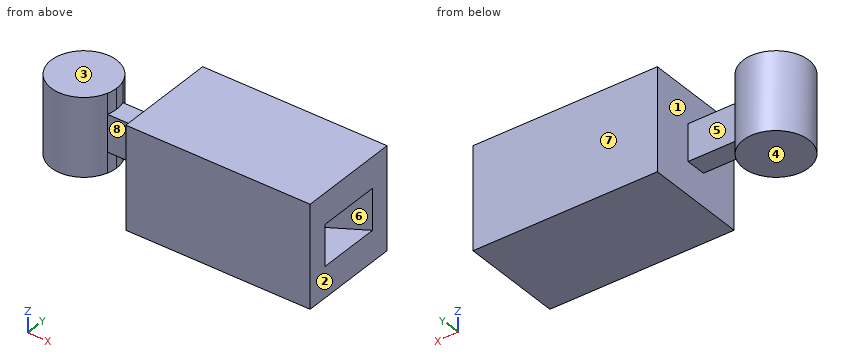
```python
from build123d import *

# Parameters (mm, degrees)
F1_DEPTH = 12.5
F2_DEPTH = 10
F3_DEPTH = 4.5
F4_DEPTH = 9.5
F5_DEPTH = 5


with BuildPart() as f1:
    # F0 (on Top) → F1 (new body, symmetric)
    with BuildSketch(Plane.XY):
        with BuildLine():
            Line((22.5, 12.5), (-22.5, 12.5))
            Line((-22.5, 12.5), (-22.5, 2.5))
            Line((-22.5, 2.5), (-22.5, -2.5))
            Line((-22.5, -2.5), (-22.5, -12.5))
            Line((-22.5, -12.5), (22.5, -12.5))
            Line((22.5, -12.5), (22.5, -7.75))
            Line((22.5, -7.75), (14.5, -3))
            ThreePointArc((14.5, -3), (-1.952987, 0), (14.5, 3))
            Line((14.5, 3), (22.5, 7.75))
            Line((22.5, 7.75), (22.5, 12.5))
        make_face()
        with BuildLine():
            ThreePointArc((15.047013, 0), (14.909142, 1.524731), (14.5, 3))
            ThreePointArc((14.5, 3), (-1.952987, 0), (14.5, -3))
            ThreePointArc((14.5, -3), (14.909142, -1.524731), (15.047013, 0))
        make_face()
        Polygon((22.5, -7.75), (22.5, -3), (14.5, -3), align=None)
        with BuildLine():
            Line((22.5, -3), (22.5, 3))
            Line((22.5, 3), (14.5, 3))
            ThreePointArc((14.5, 3), (14.909142, 1.524731), (15.047013, 0))
            ThreePointArc((15.047013, 0), (14.909142, -1.524731), (14.5, -3))
            Line((14.5, -3), (22.5, -3))
        make_face()
        Polygon((22.5, 3), (22.5, 7.75), (14.5, 3), align=None)
    extrude(amount=F1_DEPTH, both=True)

    # F0 (on Top) → F2 (cut, symmetric)
    with BuildSketch(Plane.XY):
        with BuildLine():
            ThreePointArc((15.047013, 0), (14.909142, 1.524731), (14.5, 3))
            ThreePointArc((14.5, 3), (-1.952987, 0), (14.5, -3))
            ThreePointArc((14.5, -3), (14.909142, -1.524731), (15.047013, 0))
        make_face()
    extrude(amount=F2_DEPTH, both=True, mode=Mode.SUBTRACT)

    # F0 (on Top) → F3 (join, symmetric)
    with BuildSketch(Plane.XY):
        with BuildLine():
            Line((-22.5, -2.5), (-22.5, 2.5))
            Line((-22.5, 2.5), (-34.5, 2.5))
            ThreePointArc((-34.5, 2.5), (-34.200142, 1.265951), (-34.099342, 0))
            ThreePointArc((-34.099342, 0), (-34.200142, -1.265951), (-34.5, -2.5))
            Line((-34.5, -2.5), (-22.5, -2.5))
        make_face()
    extrude(amount=F3_DEPTH, both=True)

    # F0 (on Top) → F4 (join, symmetric)
    with BuildSketch(Plane.XY):
        with BuildLine():
            ThreePointArc((-34.099342, 0), (-34.200142, 1.265951), (-34.5, 2.5))
            ThreePointArc((-34.5, 2.5), (-50.099342, 0), (-34.5, -2.5))
            ThreePointArc((-34.5, -2.5), (-34.200142, -1.265951), (-34.099342, 0))
        make_face()
    extrude(amount=F4_DEPTH, both=True)

    # F0 (on Top) → F5 (cut, symmetric)
    with BuildSketch(Plane.XY):
        Polygon((22.5, 3), (22.5, 7.75), (14.5, 3), align=None)
        with BuildLine():
            Line((22.5, -3), (22.5, 3))
            Line((22.5, 3), (14.5, 3))
            ThreePointArc((14.5, 3), (14.909142, 1.524731), (15.047013, 0))
            ThreePointArc((15.047013, 0), (14.909142, -1.524731), (14.5, -3))
            Line((14.5, -3), (22.5, -3))
        make_face()
        Polygon((22.5, -7.75), (22.5, -3), (14.5, -3), align=None)
    extrude(amount=F5_DEPTH, both=True, mode=Mode.SUBTRACT)


solid = f1.part
```
Check sheet for the modelled part. Datum: model origin and axes. Units: mm. Face numbers are marked on the shaded views. A direction names the side the tool comes from. Give positions to 0.01 mm unless a question says otherwise; leave off trailing zeros. Order: outer loops, then holes, each group sorted by start corner. A loop starts at its lowest first (then second) coordinate and runs counter-clockwise, first axis right, second up. Notation, with made-up numbers: M 82.25,59 L 91.25,59 A8 ccw 91.25,74 Z; hole C 10.25,60.5 d2. An arc over 180 degrees is marked long. Answer in a Markdown table with one row per item. Add a question column.
Q1. Access from +Z, -Z, +X, -X, +Y, -Y to the whole of each face (thin tool, end or side, straight path). Record for the marked faces 4, 5, 6, 7 and 8.
Q2. Release check for a two-part mould opening along X. For the marked faces 1, 2 and 3 record: released by +X, released by -X, zero draft, split by the parting line, or undercut.
Q3. Sectioned sample at A-A, the plane z = -7.25. Record the boundary of the cut face in (x, y), and give its area (3 significant figures).
Q4. Sectioned sample at B-B, the plane y = 4.5. Record the boundary of the cut face in (x, z), and give its area (3 significant figures).
Q5. Gauge pin test, flat ends, axial feed: pin 1 Ø6 at (y, z) = (4, 0.5) entering from +X; pin 2 Ø10 at (y, z) = (-8, -3.5) entering from -X; pin 3 Ø12.5 at (y, z) = (-3, 5) entering from -X; pin 4 Ø7 at (x, z) = (-28.5, 1) entering from +Y. Record the tip position at first contact, or that the pin passes through.
Q6. Sectioned sample at D-D, the plane x = 5. Record the boundary of the cut face in (y, z), and give its area (3 significant figures).
Q7. Sectioned sample at C-C, the plane z = 2. Record the boundary of the cut face in (x, y).
Q8. Thickness scan on L1, parallel to Z at x = 19.5, y = -4.5; L2, parallel to Z at x = -1, y = 3.5; L3, parallel to X at y = 3.5, z = 6.5. Record the ranges inside material, lowest first.
Verdict:
| question | item | result |
|---|---|---|
| 1 | face 4 | -Z, -X, +Y, -Y |
| 1 | face 5 | +Z, -Z, +Y |
| 1 | face 6 | +X |
| 1 | face 7 | +Z, -Z, +X, -X, +Y |
| 1 | face 8 | +Z, -Z, -Y |
| 2 | face 1 | undercut |
| 2 | face 2 | released by +X |
| 2 | face 3 | zero draft |
| 3 | outline | M -34.5,-2.5 A8 ccw -34.1,0 A8 ccw -34.5,2.5 A8 ccw long Z; M -22.5,-12.5 L 22.5,-12.5 L 22.5,12.5 L -22.5,12.5 Z; hole M 14.5,-3 A8.5 ccw 15.05,0 A8.5 ccw 14.5,3 A8.5 ccw long Z |
| 3 | area | 1,100 mm² |
| 4 | outline | M -48.71,-9.5 L -35.48,-9.5 L -35.48,9.5 L -48.71,9.5 Z; M -22.5,-12.5 L 22.5,-12.5 L 22.5,-5 L 17.03,-5 L 17.03,5 L 22.5,5 L 22.5,12.5 L -22.5,12.5 Z; hole M -0.66,-10 L 13.76,-10 L 13.76,10 L -0.66,10 Z |
| 4 | area | 1,030 mm² |
| 5 | pin 1 | x = 21.24 |
| 5 | pin 2 | x = -49.52 |
| 5 | pin 3 | x = -50.1 |
| 5 | pin 4 | y = 2.5 |
| 6 | outline | M -12.5,-12.5 L 12.5,-12.5 L 12.5,12.5 L -12.5,12.5 Z; hole M -8.36,-10 L 8.36,-10 L 8.36,10 L -8.36,10 Z |
| 6 | area | 291 mm² |
| 7 | outline | M -34.5,-2.5 L -22.5,-2.5 L -22.5,-12.5 L 22.5,-12.5 L 22.5,-7.75 L 14.5,-3 A8.5 cw long 14.5,3 L 22.5,7.75 L 22.5,12.5 L -22.5,12.5 L -22.5,2.5 L -34.5,2.5 A8 ccw long Z |
| 8 | L1 | -12.5 to -5, 5 to 12.5 |
| 8 | L2 | -12.5 to -10, 10 to 12.5 |
| 8 | L3 | -49.29 to -34.91, -22.5 to -1.2, 14.29 to 22.5 |
